from build123d import *

# Parameters (mm, degrees)
PAD_DEPTH     = 3.556
SKETCH001_W   = 7.239
SKETCH001_H   = 7.239
PAD001_DEPTH  = 3.81
SKETCH002_W   = 7.239
SKETCH002_H   = 7.239
PAD002_DEPTH  = 3.81
SKETCH003_R   = 1.25
HOLE_DEPTH    = 64.771
SKETCH004_R   = 0.8
HOLE001_DEPTH = 24.892


with BuildPart() as part:
    # Sketch → Pad (new body)
    with BuildSketch(Plane.XY):
        Polygon((-32.385, 0), (-32.385, -10.795), (-28.575, -10.795), (-28.575, -3.81), (28.575, -3.81), (28.575, -10.795), (32.385, -10.795), (32.385, 0), align=None)
    extrude(amount=PAD_DEPTH)

    # Sketch001 (on Face1 of Pad) → Pad001 (join)
    with BuildSketch(Plane(origin=(-32.385, 0, 0), x_dir=(0, -1, 0), z_dir=(-1, 0, 0))):
        with Locations((7.1755, -3.6195)):
            Rectangle(SKETCH001_W, SKETCH001_H)
    extrude(amount=-PAD001_DEPTH)

    # Sketch002 (on Face4 of Pad001) → Pad002 (join)
    with BuildSketch(Plane.YZ.offset(32.385)):
        with Locations((-7.1755, -3.6195)):
            Rectangle(SKETCH002_W, SKETCH002_H)
    extrude(amount=-PAD002_DEPTH)

    # Sketch003 (on Face12 of Pad002) → Hole (cut, through all)
    with BuildSketch(Plane.YZ.offset(32.385)):
        with Locations((-7.1755, -4.572)):
            Circle(SKETCH003_R)
    extrude(amount=-HOLE_DEPTH, mode=Mode.SUBTRACT)

    # Sketch004 (on Face5 of Hole) → Hole001 (cut)
    with BuildSketch(Plane.XY.offset(3.556)):
        with Locations((-8.89, -1.905)):
            Circle(SKETCH004_R)
        with Locations((8.89, -1.905)):
            Circle(SKETCH004_R)
    extrude(amount=-HOLE001_DEPTH, mode=Mode.SUBTRACT)


solid = part.part
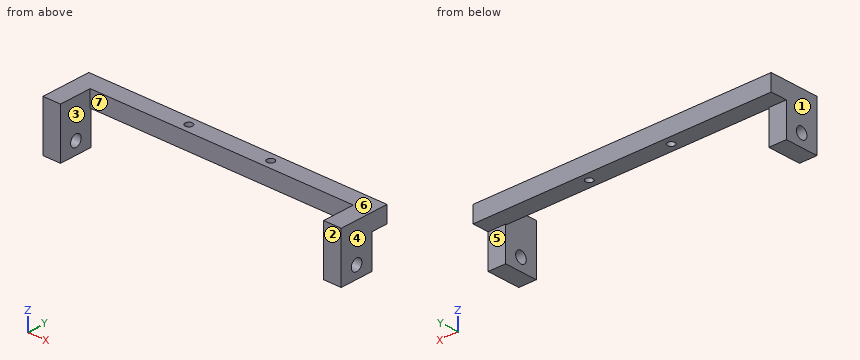
Geometry: final body of the model. Coordinates: model frame, mm. Face numbers are marked on the shaded views. A direction names the side the tool comes from. Coordinates: 2 decimals unless noted, no trailing zeros. Loops run counter-clockwise (first coordinate to the right, second up) from the corner with the lowest first, then second, coordinate; pieces in that order, holes last. Notation, with made-up numbers: M 35,27 L 79,27 A26 cw 79,58 Z; hole C 75.25,-37.75 d9. An arc over 180 degrees is marked long. One line per item, written item: value. Start each with the question number.
1) Cut plane A-A (x = 8.89). Return loops of the section in (y, z) (3 decimals), then the cut area to 3 significant figures.
2) Reachability of the marked faces 5, 6 and 7 from +Z, -Z, +X, -X, +Y, -Y: full face, straight path, thin tool, end or side. Return the list, or none.
3) Pin query (flat end, axial travel): P1, Ø2, axis at y = -7.18, z = -4.57, coming from the +X side; P2, Ø1, axis at x = 2.5, z = 2.5, coming from the +Y side; P3, Ø4, axis at x = -31, z = -3, coming from the +Y side; P4, Ø1.8, axis at x = 8.89, y = -1.905, coming from the -Z side. Return the tip coordinate at first contact, or that it passes through.
4) Draft query along X for the marked faces 1, 2, 3 and 4. Return one class per face: released by +X, released by -X, zero draft, split by the parting line, or undercut.
5) Cut plane B-B (y = -6.75). Return loops of the section in (x, z) (3 decimals).
6) Material intervals for L1, parallel to X at y = -5, z = -1.5 (3 decimals); L2, parallel to Y at x = -8.89, z = 2.45 (3 decimals); L3, parallel to Z at x = -2.5, y = -3.25, sorted ascending. Write a range as from..to.
7) Cut plane C-C (z = 1.25). Return loops of the section in (x, y) (3 decimals), then the cut area to 3 significant figures.
8) Cut plane D-D (z = -5.25). Return loops of the section in (x, y) (3 decimals), then the cut area to 3 significant figures.
Evaluation:
1. outline: M -3.81,0 L -2.705,0 L -2.705,3.556 L -3.81,3.556 Z; M -1.105,0 L 0,0 L 0,3.556 L -1.105,3.556 Z
1. area: 7.86 mm^2
2. face 5: -Z, +X, -X, +Y
2. face 6: +Z, +X, -X, +Y, -Y
2. face 7: +Z, -Z, -Y
3. P1: through
3. P2: y = 0
3. P3: y = -3.56
3. P4: z = 0
4. face 1: released by -X
4. face 2: zero draft
4. face 3: undercut
4. face 4: released by +X
5. outline: M -32.385,-7.239 L -28.575,-7.239 L -28.575,-5.747 L -32.385,-5.747 Z; M -32.385,-3.397 L -28.575,-3.397 L -28.575,3.556 L -32.385,3.556 Z; M 28.575,-7.239 L 32.385,-7.239 L 32.385,-5.747 L 28.575,-5.747 Z; M 28.575,-3.397 L 32.385,-3.397 L 32.385,3.556 L 28.575,3.556 Z
6. L1: -32.385..-28.575, 28.575..32.385
6. L2: -3.81..-2.705, -1.105..0
6. L3: 0..3.56
7. outline: M -32.385,-10.795 L -28.575,-10.795 L -28.575,-3.81 L 28.575,-3.81 L 28.575,-10.795 L 32.385,-10.795 L 32.385,0 L -32.385,0 Z; hole C -8.89,-1.905 d1.6; hole C 8.89,-1.905 d1.6
7. area: 296 mm^2
8. outline: M -32.385,-10.795 L -28.575,-10.795 L -28.575,-8.226 L -32.385,-8.226 Z; M -32.385,-6.125 L -28.575,-6.125 L -28.575,-3.556 L -32.385,-3.556 Z; M 28.575,-10.795 L 32.385,-10.795 L 32.385,-8.226 L 28.575,-8.226 Z; M 28.575,-6.125 L 32.385,-6.125 L 32.385,-3.556 L 28.575,-3.556 Z
8. area: 39.2 mm^2
